For this review, take the finished solid that the model builds, in its own axes (mm). Face numbers are marked on the shaded views. Round coordinates to 2 decimals unless told otherwise and drop trailing zeros. Write each loop counter-clockwise with the first axis right and the second up, starting at its lowest first coordinate (ties: lowest second). Pieces come first, ordered by that corner, then holes. Notation, with made-up numbers: (49, -3.5) -> (67, -3.5) arc R25 cw to (67, 31.5) -> close; hole circle Ø1 at (76.5, 38.25). An arc over 180 degrees is marked (long way). Answer in a Markdown table with one row per item. Add a question column.
```python
from build123d import *

# Parameters (mm, degrees)
F0_R     = 30
F1_DEPTH = 17.5
F0_R_2   = 41.85
F0_R_3   = 40.25
F2_DEPTH = 12
F3_DEPTH = 0.15
F4_R     = 3
F5_R     = 8


with BuildPart() as f1:
    # F0 (on Top) → F1 (new body)
    with BuildSketch(Plane.XY):
        Circle(F0_R)
    extrude(amount=F1_DEPTH)

    # F0 (on Top) → F2 (join)
    with BuildSketch(Plane.XY):
        Circle(F0_R_2)
        Circle(F0_R_3, mode=Mode.SUBTRACT)
        Circle(F0_R_3)
        Circle(F0_R, mode=Mode.SUBTRACT)
    extrude(amount=F2_DEPTH)

    # F0 (on Top) → F3 (cut)
    with BuildSketch(Plane.XY):
        Circle(F0_R_3)
        Circle(F0_R, mode=Mode.SUBTRACT)
        Circle(F0_R)
    extrude(amount=F3_DEPTH, mode=Mode.SUBTRACT)

    # F4
    f4_edges = [f1.edges().sort_by_distance(p)[0] for p in [
        (-30, 0, 17.5),
    ]]
    fillet(f4_edges, radius=F4_R)

    # F5
    f5_edges = [f1.edges().sort_by_distance(p)[0] for p in [
        (-41.85, 0, 12),
    ]]
    fillet(f5_edges, radius=F5_R)


solid = f1.part
```
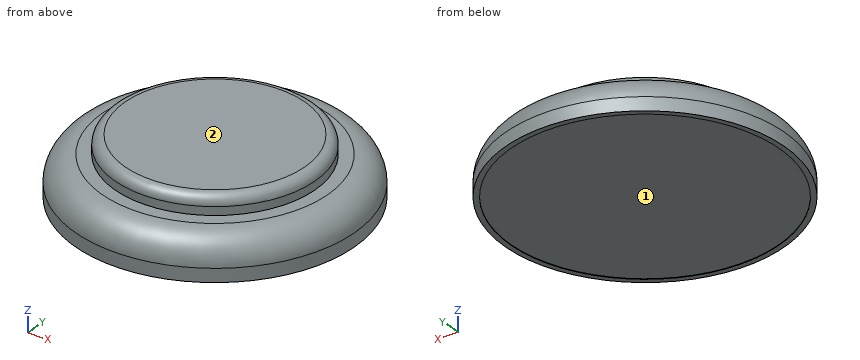
1. For L1, parallel to Y at x = 0, z = 0.1; L2, parallel to Z at x = 5.5, y = 3; L3, parallel to Z at x = -13, y = -31.5, list the stretches that pass through material, from the lowest coordinate up. Write a range as [from, to].
2. Clearance check with flat-ended pins moving along their axes: pin 1 Ø4 at (y, z) = (30, 12) entering from +X; pin 2 Ø1.5 at (y, z) = (-21.5, 9) entering from +X; pin 3 Ø4 at (y, z) = (25, 5) entering from +X. State where each tip first meets the part, or that it passes through.
3. We need section A-A (x = 0). Write out the cut boundary in (y, z), plus the area to 3 significant figures.
4. The part is to be moulded in two halves that separate along Y. For the marked faces 1 and 2, say which applies: pulls with the +Y half, pulls with the -Y half, needs draft (parallel to the pull), parting line crosses it, or undercut.
5. We need section C-C (z = 5.5). Write out the cut boundary in (x, y), plus the area to 4 significant figures.
Response:
| question | item | result |
|---|---|---|
| 1 | L1 | [-41.85, -40.25], [40.25, 41.85] |
| 1 | L2 | [0.15, 17.5] |
| 1 | L3 | [0.15, 12] |
| 2 | pin 1 | x = 25.81 |
| 2 | pin 2 | x = 34.64 |
| 2 | pin 3 | x = 34.91 |
| 3 | outline | (-41.85, 0) -> (-40.25, 0) -> (-40.25, 0.15) -> (40.25, 0.15) -> (40.25, 0) -> (41.85, 0) -> (41.85, 4) arc R8 ccw to (33.85, 12) -> (30, 12) -> (30, 14.5) arc R3 ccw to (27, 17.5) -> (-27, 17.5) arc R3 ccw to (-30, 14.5) -> (-30, 12) -> (-33.85, 12) arc R8 ccw to (-41.85, 4) -> close |
| 3 | area | 1,290 mm2 |
| 4 | face 1 | undercut |
| 4 | face 2 | needs draft |
| 5 | outline | circle Ø83.42 at (0, 0) |
| 5 | area | 5,465 mm2 |
